```python
from build123d import *

# Parameters (mm, degrees)
BOSS_EXTRUDE1_DEPTH      = 320
BOSS_EXTRUDE1_DEPTH_BACK = 320
LPATTERN2_COUNT          = 11
LPATTERN2_PITCH          = 60
CHAMFER1_SIZE            = 0.5
CUT_EXTRUDE1_DEPTH       = 321.661815625
CUT_EXTRUDE1_DEPTH_BACK  = 321.661815625


with BuildPart() as part:
    # Sketch3 → Boss-Extrude1 (new, two sides: drawn at the far end of the back side and taken through both)
    with BuildSketch(Plane.XY.offset(-BOSS_EXTRUDE1_DEPTH_BACK)):
        with BuildLine():
            Line((3, 9), (-3, 9))
            Line((-3, 9), (-7.160036564, 9))
            Line((-7.160036564, 9), (-7.767930373, 8.392105714))
            ThreePointArc((-7.767930373, 8.392105714), (-8.344874488, 7.264307267), (-9.472673258, 6.687363783))
            Line((-9.472673258, 6.687363783), (-10, 6.160037041))
            Line((-10, 6.160037041), (-10, 4.82918644))
            Line((-10, 4.82918644), (-9.472673258, 4.314376637))
            ThreePointArc((-9.472673258, 4.314376637), (-8.341068744, 3.731631743), (-7.767930373, 2.595131504))
            Line((-7.767930373, 2.595131504), (-6.550048828, 1.379235268))
            Line((-6.550048828, 1.379235268), (-6.550048828, -1.550048828))
            Line((-6.550048828, -1.550048828), (-10, -4.999922752))
            Line((-10, -4.999922752), (-10, -8))
            Line((-10, -8), (-9, -9))
            Line((-9, -9), (0, -9))
            Line((0, -9), (9, -9))
            Line((9, -9), (10, -8))
            Line((10, -8), (10, -4.999922752))
            Line((10, -4.999922752), (6.550048828, -1.550048828))
            Line((6.550048828, -1.550048828), (6.550048828, 1.379235268))
            Line((6.550048828, 1.379235268), (7.767930373, 2.595131504))
            ThreePointArc((7.767930373, 2.595131504), (8.341068744, 3.731631743), (9.472673258, 4.314376637))
            Line((9.472673258, 4.314376637), (10, 4.82918644))
            Line((10, 4.82918644), (10, 6.160037041))
            Line((10, 6.160037041), (9.472673258, 6.687363783))
            ThreePointArc((9.472673258, 6.687363783), (8.344874488, 7.264307267), (7.767930373, 8.392105714))
            Line((7.767930373, 8.392105714), (7.160036564, 9))
            Line((7.160036564, 9), (3, 9))
        make_face()
    extrude(amount=BOSS_EXTRUDE1_DEPTH + BOSS_EXTRUDE1_DEPTH_BACK)

    # Sketch4 → Cut-Revolve1 (revolve, cut)
    with BuildSketch(Plane(origin=(0, 0, 0), x_dir=(0, 0, -1), z_dir=(1, 0, 0)), mode=Mode.PRIVATE) as cut_revolve1_sk:
        Polygon((-295.25, 9), (-300, 9), (-300, -9), (-297, -9), (-297, 0.5), (-295.25, 0.5), align=None)
    cut_revolve1 = revolve(cut_revolve1_sk.sketch.rotate(Axis((0, 9, 300), (0, -1, 0)), 180), axis=Axis((0, 9, 300), (0, -1, 0)), mode=Mode.SUBTRACT)

    # LPattern2: Cut-Revolve1 ×11
    with Locations(*[(0, 0, -i * LPATTERN2_PITCH) for i in range(1, LPATTERN2_COUNT)]):
        add(cut_revolve1, mode=Mode.SUBTRACT)

    # Chamfer1
    chamfer1_edges = [part.edges().sort_by_distance(p)[0] for p in [
        (-6.550048828, -0.08540678, 320),
        (-8.275024414, -3.27498579, 320),
        (-10, -6.499961376, 320),
        (-9.5, -8.5, 320),
        (0, -9, 320),
        (9.5, -8.5, 320),
        (10, -6.499961376, 320),
        (8.275024414, -3.27498579, 320),
        (6.550048828, -0.08540678, 320),
        (-8.341068744, 3.731631743, 320),
        (7.158989601, 1.987183386, 320),
        (8.341068744, 3.731631743, 320),
        (9.736336629, 4.571781538, 320),
        (-9.736336629, 4.571781538, -320),
        (-10, 5.49461174, -320),
        (10, 5.49461174, 320),
        (-9.736336629, 6.423700412, -320),
        (-7.463983469, 8.696052857, -320),
        (0, 9, -320),
        (7.463983469, 8.696052857, -320),
        (9.736336629, 6.423700412, -320),
        (10, 5.49461174, -320),
        (9.736336629, 6.423700412, 320),
        (9.736336629, 4.571781538, -320),
        (7.158989601, 1.987183386, -320),
        (6.550048828, -0.08540678, -320),
        (8.275024414, -3.27498579, -320),
        (10, -6.499961376, -320),
        (9.5, -8.5, -320),
        (0, -9, -320),
        (8.344874488, 7.264307267, 320),
        (-9.5, -8.5, -320),
        (-10, -6.499961376, -320),
        (-8.275024414, -3.27498579, -320),
        (-6.550048828, -0.08540678, -320),
        (-7.158989601, 1.987183386, -320),
        (-8.341068744, 3.731631743, -320),
        (-8.344874488, 7.264307267, -320),
        (8.344874488, 7.264307267, -320),
        (8.341068744, 3.731631743, -320),
        (7.463983469, 8.696052857, 320),
        (0, 9, 320),
        (-7.463983469, 8.696052857, 320),
        (-8.344874488, 7.264307267, 320),
        (-7.158989601, 1.987183386, 320),
        (-9.736336629, 6.423700412, 320),
        (-10, 5.49461174, 320),
        (-9.736336629, 4.571781538, 320),
    ]]
    chamfer(chamfer1_edges, length=CHAMFER1_SIZE)

    # Sketch7 → Cut-Extrude1 (cut, two sides: drawn at the far end of the back side and taken through both)
    with BuildSketch(Plane.XZ.offset(9).offset(-CUT_EXTRUDE1_DEPTH_BACK)):
        Polygon((1255.011383847, 289.6), (23.92488735, 289.6), (-18.541494628, 289.6), (-1249.627991125, 289.6), (-1249.627991125, 2751.772992994), (1255.011383847, 2751.772992994), align=None)
    extrude(amount=CUT_EXTRUDE1_DEPTH + CUT_EXTRUDE1_DEPTH_BACK, mode=Mode.SUBTRACT)


solid = part.part
```
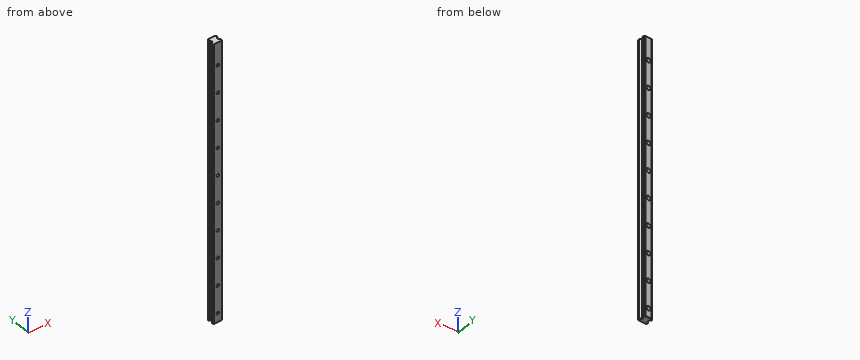
For this review, take the finished solid that the model builds, in its own axes (mm). Give positions to 0.01 mm unless a question says otherwise; leave off trailing zeros. Write each loop counter-clockwise with the first axis right and the second up, starting at its lowest first coordinate (ties: lowest second). Pieces come first, ordered by that corner, then holes. Notation, with made-up numbers: M -3.75,4.5 L 34.25,4.5 A19 cw 34.25,17.5 Z; hole C 31,1 d5. An arc over 180 degrees is marked long. Answer as a JSON object with one key per item and string values. Group by question number.
Item 1: For pin 1 Ø4 at (y, z) = (-2.5, 137) entering from -X; pin 2 Ø3.5 at (x, z) = (0, 0) entering from -Y; pin 3 Ø3 at (y, z) = (-2, -239) entering from -X; pin 4 Ø1.5 at (y, z) = (-0.5, 89.5) entering from -X, all flat-tipped, find the tip position at first contact; note any pin that passes through.
Item 2: For probe 1 along X at (y, z) = (8.25, 233); probe 2 along Y at (x, z) = (6.75, 260.5); probe 3 along X at (y, z) = (1.25, 218), list the stretches that pass through material, from the lowest coordinate up. Write a range as [from, to].
Item 3: Consider section A-A on z = 14.5. Write out the cut boundary in (x, y), plus the area to 3 significant figures.
Check result:
{
 "1": {"pin 1": "stops at x = -9.5", "pin 2": "passes through", "pin 3": "stops at x = -8.5", "pin 4": "stops at x = -6.55"},
 "2": {"probe 1": "x = [-7.8, 7.8]", "probe 2": "y = [-9, -1.75], [1.58, 9]", "probe 3": "x = [-6.55, 6.55]"},
 "3": {"outline": "M -10,-8 L -9,-9 L 9,-9 L 10,-8 L 10,-5 L 6.55,-1.55 L 6.55,1.38 L 7.77,2.6 A2.06 cw 9.47,4.31 L 10,4.83 L 10,6.16 L 9.47,6.69 A2.06 cw 7.77,8.39 L 7.16,9 L -7.16,9 L -7.77,8.39 A2.06 cw -9.47,6.69 L -10,6.16 L -10,4.83 L -9.47,4.31 A2.06 cw -7.77,2.6 L -6.55,1.38 L -6.55,-1.55 L -10,-5 Z", "area": "304 mm^2"}
}
